Build history of the part. All positions in model axes, mm. A direction names the side the tool comes from. Coordinates: 2 decimals unless noted, no trailing zeros. One line per item, written item: value.
from build123d import *

# Parameters (mm, degrees)
SKIZZE1_W                       = 40
SKIZZE1_H                       = 40
AUFSATZ_LINEAR_AUSTRAGEN1_DEPTH = 66
M4_GEWINDEBOHRUNG1_D            = 3.3
M4_GEWINDEBOHRUNG1_DEPTH        = 11.5
M4_GEWINDEBOHRUNG1_TIP          = 0.991420021
M6_GEWINDEBOHRUNG1_D            = 5
M6_GEWINDEBOHRUNG1_DEPTH        = 17
M6_GEWINDEBOHRUNG1_CSINK_D      = 6.05
M6_GEWINDEBOHRUNG1_CSINK_ANGLE  = 90
M6_GEWINDEBOHRUNG1_TIP          = 1.502151548
F_6_0MM_STIFTLOCH1_D            = 6
F_6_0MM_STIFTLOCH1_DEPTH        = 17
F_6_0MM_STIFTLOCH1_TIP          = 1.802581857


with BuildPart() as part:
    # Skizze1 → Aufsatz-Linear austragen1 (new, symmetric)
    with BuildSketch(Plane(origin=(0, 0, 0), x_dir=(1, 0, 0), z_dir=(0, 1, 0))):
        Rectangle(SKIZZE1_W, SKIZZE1_H)
    extrude(amount=AUFSATZ_LINEAR_AUSTRAGEN1_DEPTH, both=True)

    # M4 Gewindebohrung1
    with Locations(Plane(origin=(0, 66, 0), x_dir=(1, 0, 0), z_dir=(0, 1, 0))):
        with Locations((-12.5, 12.5), (12.5, 12.5), (12.5, -12.5), (-12.5, -12.5)):
            Hole(M4_GEWINDEBOHRUNG1_D / 2, depth=M4_GEWINDEBOHRUNG1_DEPTH)
            with Locations((0, 0, -(M4_GEWINDEBOHRUNG1_DEPTH + M4_GEWINDEBOHRUNG1_TIP / 2))):  # 118° drill point
                Cone(0, M4_GEWINDEBOHRUNG1_D / 2, M4_GEWINDEBOHRUNG1_TIP, mode=Mode.SUBTRACT)

    # M6 Gewindebohrung1
    with Locations(Plane(origin=(0, -66, 0), x_dir=(-1, 0, 0), z_dir=(0, -1, 0))):
        with Locations((10, 12.5), (10, -12.5)):
            CounterSinkHole(M6_GEWINDEBOHRUNG1_D / 2, M6_GEWINDEBOHRUNG1_CSINK_D / 2, depth=M6_GEWINDEBOHRUNG1_DEPTH, counter_sink_angle=M6_GEWINDEBOHRUNG1_CSINK_ANGLE)
            with Locations((0, 0, -(M6_GEWINDEBOHRUNG1_DEPTH + M6_GEWINDEBOHRUNG1_TIP / 2))):  # 118° drill point
                Cone(0, M6_GEWINDEBOHRUNG1_D / 2, M6_GEWINDEBOHRUNG1_TIP, mode=Mode.SUBTRACT)

    # Ø6.0mm Stiftloch1
    with Locations(Plane(origin=(0, -66, 0), x_dir=(-1, 0, 0), z_dir=(0, -1, 0))):
        with Locations((10, 0), (-10, 0)):
            Hole(F_6_0MM_STIFTLOCH1_D / 2, depth=F_6_0MM_STIFTLOCH1_DEPTH)
            with Locations((0, 0, -(F_6_0MM_STIFTLOCH1_DEPTH + F_6_0MM_STIFTLOCH1_TIP / 2))):  # 118° drill point
                Cone(0, F_6_0MM_STIFTLOCH1_D / 2, F_6_0MM_STIFTLOCH1_TIP, mode=Mode.SUBTRACT)


solid = part.part
1. Flat gauge pins, fed straight in: P1, Ø2, axis at x = -12.5, z = 12.5, coming from the +Y side; P2, Ø2.5, axis at x = 12.5, z = 12.5, coming from the +Y side; P3, Ø6, axis at x = -10, z = -12.5, coming from the -Y side (3 decimals). Where does each tip first touch, or does it go through?
Values found:
P1: stops at y = 54.11
P2: stops at y = 54.26
P3: stops at y = -65.975
2. 3-axis set-ups, long thin cutter, end or side, ignore diameter. For faces 1 (the face through (0, 1, 20)), 2 (the face through (-12.4, -57.4, 1.8)), 3 (the face through (10.976, 60.17, 13.132)): which of +Z, -Z, +X, -X, +Y, -Y reach the whole face in a straight line?
Values found:
face 1: +Z, +X, -X, +Y, -Y
face 2: -Y
face 3: +Y
3. Probe line 1 along Z through (x, y) = (-10, -55.5); line 2 along X through (y, z) = (60, -12.5). List the from-to ranges inside material, lowest first.
Values found:
line 1: z = -20 to -15, -10 to -3, 3 to 10, 15 to 20
line 2: x = -20 to -14.15, -10.85 to 10.85, 14.15 to 20
4. Two-plate mould, pull along X, no slides. Class faces 4 (the face through (0, 1, -20)), 5 (the face through (20, 1, 0)), 6 (the face through (-9.68, -47.759, -12.793)): pulls with the +X half, pulls with the -X half, needs draft (parallel to the pull), parting line crosses it, or undercut.
Values found:
face 4: needs draft
face 5: pulls with the +X half
face 6: undercut
